Part model, mm, in its own coordinate system. Face numbers are marked on the shaded views. A direction names the side the tool comes from. Round coordinates to 2 decimals unless told otherwise and drop trailing zeros. Loops run counter-clockwise (first coordinate to the right, second up) from the corner with the lowest first, then second, coordinate; pieces in that order, holes last. Notation, with made-up numbers: M 59.25,42 L 118.25,42 A15 cw 118.25,68 Z; hole C 31.25,-15 d2. An arc over 180 degrees is marked long. Put each result on its own line as item: value. Start each with the question number.
1) Slice it at B-B on x = 31. Give the cut face in (y, z), then the cut area to 3 significant figures.
2) Slice it at C-C on z = 7.5. Give the cut face in (x, y).
3) Slice it at D-D on y = 3. Give the cut face in (x, z), then the cut area to 3 significant figures.
4) Which spindle directions (+Z, -Z, +X, -X, +Y, -Y) get a long thin tool onto all of the face, cutting with end or side? Do the marked faces 1 and 2. Say none if no direction does.
5) Drop a flat-ended pin along its axis: pin 1 Ø1 at (x, y) = (123, 27.5) entering from +Z. Give the stop position or say it passes through.
6) Slice it at A-A on y = 12. Give the cut face in (x, z), then the cut area to 3 significant figures.
7) Probe line 1 along Y through (x, z) = (-1.25, 26.5); line 2 along X through (y, z) = (11.5, 33); line 3 along Z through (x, y) = (-1.25, 12). List the from-to ranges inside material, lowest first.
Autodesk Inventor part; units mm, degrees
ref_plane "YZ Plane" through (0, 0, 0) normal (1, 0, 0) x (0, 1, 0)
ref_plane "XZ Plane" through (0, 0, 0) normal (0, 1, 0) x (-1, 0, 0)
ref_plane "XY Plane" through (0, 0, 0) normal (0, 0, 1) x (1, 0, 0)
sketch "Sketch1" plane through (0, 0, 0) normal (0, 0, 1) x (1, 0, 0)
  line L0 (0, 44) -> (161, 44)
  line L1 (161, 44) -> (161, 0)
  line L2 (161, 0) -> (0, 0)
  line L3 (0, 0) -> (0, 44)
  dimension "d0" = 161
  dimension "d1" = 44
extrude "Plate1" add sketch "Sketch1" along normal blind 2
sketch "Sketch2" plane through (0, 0, 2) normal (-1, 0, 0) x (0, -1, 0)
  line L0 (-44, 0) -> (0, 0)
  line L1 (0, 0) -> (0, 50)
  line L2 (0, 50) -> (-44, 50)
  line L3 (-44, 50) -> (-44, 0)
edge flange "Flange1" height 52 angle 90 thickness 2 bend radius 2 thickness toward (-1, 0, 0) relief tear relief width 2 relief depth 1 corner gap 2 corner form 0 edges at (0, 22, 2) (161, 22, 2) wall of the first edge with corners at (0, 44, 2) (0, 0, 2) (0, 0, 52) (0, 44, 52)
bend "Bend1"
corner "Corner1"
sketch "Sketch3" plane through (163, 0, 52) normal (1, 0, 0) x (0, 0, -1)
  line L0 (0, 0) -> (0, 44) construction
  line L1 (5.5, 32) -> (5.5, 12) construction
  point P0 (52, 0)
  point P1 (25.5, 32)
  point P2 (25.5, 12)
  point P3 (0, 22)
  point P4 (5.5, 22)
  dimension "d13" = 20
  dimension "d14" = 20
  dimension "d15" = 5.5
hole "Hole1" at (163, 32, 46.5) at (163, 32, 26.5) at (163, 12, 46.5) at (163, 12, 26.5) direction (-1, 0, 0) diameter 3.4 end through all
fillet "Corner Round1" radius 6 4 edges at (-1, 0, 52) (-1, 44, 52) (162, 0, 52) (162, 44, 52)
sketch "Sketch4" plane through (0, 0, 0) normal (0, 0, -1) x (-1, 0, 0)
  line L0 (-163, 0) -> (-163, 44)
  line L1 (2, 44) -> (2, 0)
  point P0 (0, 0)
  point P1 (-130, 22)
  point P2 (-85.5, 22)
  point P3 (-75.5, 22)
  point P4 (-31, 22)
  point P5 (-163, 22)
  dimension "d24" = 10
  dimension "d25" = 33
  dimension "d26" = 33
  dimension "d27" = 44.5
  dimension "d28" = 44.5
hole "Hole2" at (130, 22, 0) at (85.5, 22, 0) at (75.5, 22, 0) at (31, 22, 0) direction (0, 0, 1) diameter 3.4 end through all
equation "\"d21\" = Thickness"
equation "\"d2\" = Thickness"
equation "\"d3\" = BendReliefWidth"
equation "\"d4\" = BendReliefDepth"
equation "\"d5\" = MinimumRemnant"
equation "\"d6\" = TransitionRadius"
equation "\"d9\" = BendRadius"
equation "\"d10\" = CornerReliefSize"
equation "\"d11\" = GapSize"
equation "\"d12\" = JacobiRadiusSize"
equation "\"BendRadius\" = Thickness"
equation "\"BendReliefWidth\" = Thickness"
equation "\"BendReliefDepth\" = 0.5 * Thickness"
equation "\"CornerReliefSize\" = 4 * Thickness"
equation "\"MinimumRemnant\" = 2 * Thickness"
equation "\"TransitionRadius\" = BendRadius"
equation "\"JacobiRadiusSize\" = BendRadius"
equation "\"GapSize\" = Thickness"
properties part number "NEW Z Bracket"
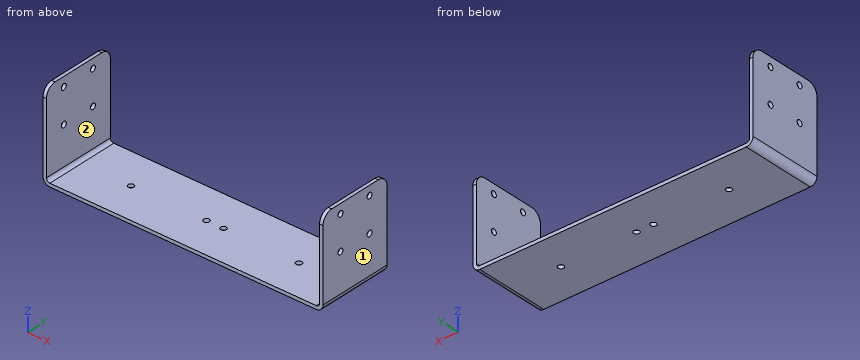
Recorded:
1. outline: M 0,0 L 20.3,0 L 20.3,2 L 0,2 Z; M 23.7,0 L 44,0 L 44,2 L 23.7,2 Z
1. area: 81.2 mm2
2. outline: M -2,0 L 0,0 L 0,44 L -2,44 Z; M 161,0 L 163,0 L 163,44 L 161,44 Z
3. outline: M -2,4 A4 ccw 2,0 L 159,0 A4 ccw 163,4 L 163,51.2 L 161,51.2 L 161,4 A2 cw 159,2 L 2,2 A2 cw 0,4 L 0,51.2 L -2,51.2 Z
3. area: 522 mm2
4. face 1: +Z, -Z, +X, +Y, -Y
4. face 2: +Z, +Y, -Y
5. pin 1: stops at z = 2
6. outline: M -2,4 A4 ccw 2,0 L 159,0 A4 ccw 163,4 L 163,24.8 L 161,24.8 L 161,4 A2 cw 159,2 L 2,2 A2 cw 0,4 L 0,24.8 L -2,24.8 Z; M -2,28.2 L 0,28.2 L 0,44.8 L -2,44.8 Z; M -2,48.2 L 0,48.2 L 0,52 L -2,52 Z; M 161,28.2 L 163,28.2 L 163,44.8 L 161,44.8 Z; M 161,48.2 L 163,48.2 L 163,52 L 161,52 Z
6. area: 498 mm2
7. line 1: y = 0 to 10.3, 13.7 to 30.3, 33.7 to 44
7. line 2: x = -2 to 0, 161 to 163
7. line 3: z = 1.67 to 24.8, 28.2 to 44.8, 48.2 to 52
